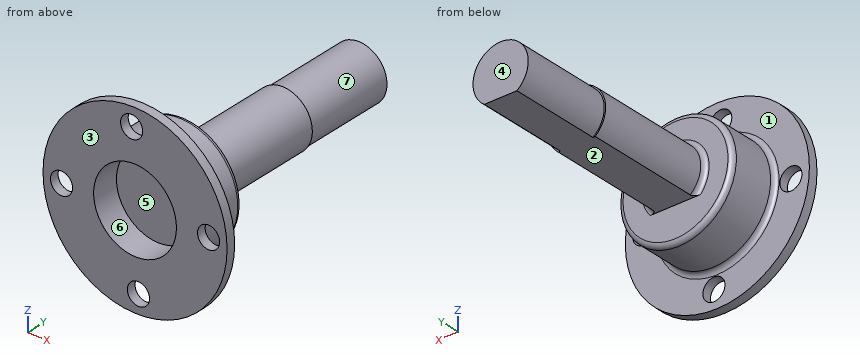
```python
from build123d import *

# Parameters (mm, degrees)
ESQUISSE3_W                  = 6.57785754
ESQUISSE3_H                  = 1.386048805
ENL_V_MAT_EXTRU_1_DEPTH      = 23
D_GAGEMENT_M21_D             = 2.4
D_GAGEMENT_M21_DEPTH         = 1.001
R_P_TITION_CIRCULAIRE1_COUNT = 4
FILLET1_R                    = 0.5


with BuildPart() as part:
    # Esquisse2 → Révolution2 (revolve)
    with BuildSketch(Plane.XY):
        Polygon((0, 29.5), (3, 29.5), (3, 19.5), (3.15, 19.5), (3.15, 6.5), (6.2, 6.5), (6.2, 3), (6.2, 1), (10, 1), (10, 0), (4.5, 0), (4.5, 3), (0, 3), align=None)
    revolve(axis=Axis((0, 3, 0), (0, 1, 0)))

    # Esquisse3 → Enlèv. mat.-Extru.1 (cut)
    with BuildSketch(Plane(origin=(0, 29.5, 0), x_dir=(1, 0, 0), z_dir=(0, 1, 0))):
        with Locations((-0.352413472, 3.114928535)):
            Rectangle(ESQUISSE3_W, ESQUISSE3_H)
    extrude(amount=-ENL_V_MAT_EXTRU_1_DEPTH, mode=Mode.SUBTRACT)

    # Dégagement M21
    with Locations(Plane(origin=(0, 1, 0), x_dir=(1, 0, 0), z_dir=(0, 1, 0))):
        with Locations((0.371303159, 7.991378727)):
            d_gagement_m21 = Hole(D_GAGEMENT_M21_D / 2, depth=D_GAGEMENT_M21_DEPTH)

    # Répétition circulaire1: Dégagement M21 ×4 about axis
    r_p_tition_circulaire1_axis = Axis((0, 0, 0), (0, 1, 0))
    for i in range(1, R_P_TITION_CIRCULAIRE1_COUNT):
        add(d_gagement_m21.rotate(r_p_tition_circulaire1_axis, i * 360 / R_P_TITION_CIRCULAIRE1_COUNT), mode=Mode.SUBTRACT)

    # Fillet1
    fillet1_edges = [part.edges().sort_by_distance(p)[0] for p in [
        (-6.2, 1, 0),
        (-6.2, 6.5, 0),
        (0, 6.5, 3.15),
    ]]
    fillet(fillet1_edges, radius=FILLET1_R)


solid = part.part
```
Could you check a few things on this model? Use its own coordinates, in mm. Face numbers are marked on the shaded views. A direction names the side the tool comes from. Coordinates: 2 decimals unless noted, no trailing zeros. Write each loop counter-clockwise with the first axis right and the second up, starting at its lowest first coordinate (ties: lowest second). Pieces come first, ordered by that corner, then holes. Notation, with made-up numbers: (71, 37.5) - (85, 37.5) arc R25 cw to (85, 49.5) - close; hole circle Ø3 at (40, -27). An arc over 180 degrees is marked (long way). Use a Markdown table: item, result.
Q1. I'm going to push flat-ended pins straight in: pin 1 Ø1 at (x, z) = (1, 2) entering from -Y; pin 2 Ø1 at (x, z) = (-7, -7) entering from +Y; pin 3 Ø10 at (y, z) = (18.5, -4.5) entering from +X. Where does each tip first touch, or does it pass through?
Geometry check:
| item | result |
|---|---|
| pin 1 | stops at y = 3 |
| pin 2 | stops at y = 1 |
| pin 3 | stops at x = 3.15 |
Q2. Thinking about a two-plate mould opening in Z: for the marked faces 4, 5, 6 and 7, which applies, +Z half, -Z half, draft (parallel to the pull), parting line (faces both ways), or undercut?
Geometry check:
| item | result |
|---|---|
| face 4 | draft |
| face 5 | undercut |
| face 6 | undercut |
| face 7 | parting line |
Q3. Imagine slicing it at D-D (y = 2.5). List the corners of the cut face in (x, z) for me, and give its area (3 significant figures).
Geometry check:
| item | result |
|---|---|
| outline | circle Ø12.4 at (0, 0); hole circle Ø9 at (0, 0) |
| area | 57.1 mm2 |
Q4. Which directions (+Z, -Z, +X, -X, +Y, -Y) give clear straight access to the entire face, cutting with the end or side of a thin tool? Please do the marked faces 1, 2 and 3.
Geometry check:
| item | result |
|---|---|
| face 1 | +Y |
| face 2 | -Z, +X, -X, +Y |
| face 3 | +Z, -Z, +X, -X, -Y |
Q5. Please list where these lines run through material, in increasing order: L1, parallel to X at y = 1.45, z = 0; L2, parallel to X at y = 0.65, z = 0; L3, parallel to Y at x = 9.25, z = -3.
Geometry check:
| item | result |
|---|---|
| L1 | x = -6.2 to -4.5, 4.5 to 6.2 |
| L2 | x = -10 to -9.13, -6.85 to -4.5, 4.5 to 6.85, 9.13 to 10 |
| L3 | y = 0 to 1 |
Q6. Imagine slicing it at A-A (x = 0). Count the separate pieces of the cut face and the enclosed holes in it, and give its area (3 significant figures).
Geometry check:
| item | result |
|---|---|
| separate pieces | 3 |
| enclosed holes | 0 |
| area | 183 mm2 |
Q7. Imagine slicing it at C-C (x = -7.5). List the corners of the cut face in (y, z) for me, and give its area (3 significant figures).
Geometry check:
| item | result |
|---|---|
| outline | (0, -6.61) - (1, -6.61) - (1, -1.47) - (0, -1.47) - close; (0, 0.72) - (1, 0.72) - (1, 6.61) - (0, 6.61) - close |
| area | 11.0 mm2 |
